The figure shows three views and two pictorial views of one solid part (mm, origin at its lowest corner). Answer the questions. A direction names the side the tool comes from. Give positions to 0.01 mm unless a question says otherwise; leave off trailing zeros. Order: outer loops, then holes, each group sorted by start corner. A loop starts at its lowest first (then second) coordinate and runs counter-clockwise, first axis right, second up. Notation, with made-up numbers: (16, 1.5) - (46, 1.5) arc R22 ccw to (46, 12.5) - close; hole circle Ø9 at (-3, -0.5). An arc over 180 degrees is marked (long way). Answer as CSV lines item,"result". Start each with the question number.
1. Section A-A on x = 170 is taken. Give the vertices of the cut face in (y, z), and give its area (3 significant figures).
2. Section D-D on y = 15.5 is taken. Give the vertices of the cut face in (x, z).
3. Section C-C on z = 8 is taken. Give the vertices of the cut face in (x, y).
4. Section B-B on y = 38.1 is taken. Give the vertices of the cut face in (x, z), and give its area (3 significant figures).
5. Which of the six approach directions +Z, -Z, +X, -X, +Y, -Y give full straight-line access (tool end or side, diameter ignored) to the marked faces 1, 2 and 3?
6. Determine the mould class of the marked faces 4, 5 and 6 for opening direction Z: +Z half, -Z half, draft (parallel to the pull), parting line (faces both ways), or undercut.
7. A flat-ended cylindrical pin translates along its axis: pin 1 (5 mm diameter, centred on y = 23, z = 61.5, fed in from +X). Find the tip coordinate at first contact, or state that the pin passes through.
8. Consider line 1 along Y through (x, z) = (170, 11); line 2 along Z through (x, y) = (84, 15.5); line 3 along X through (y, z) = (38, 86). Determine where each line is inside the solid, lowest interval first. Write a range as [from, to].
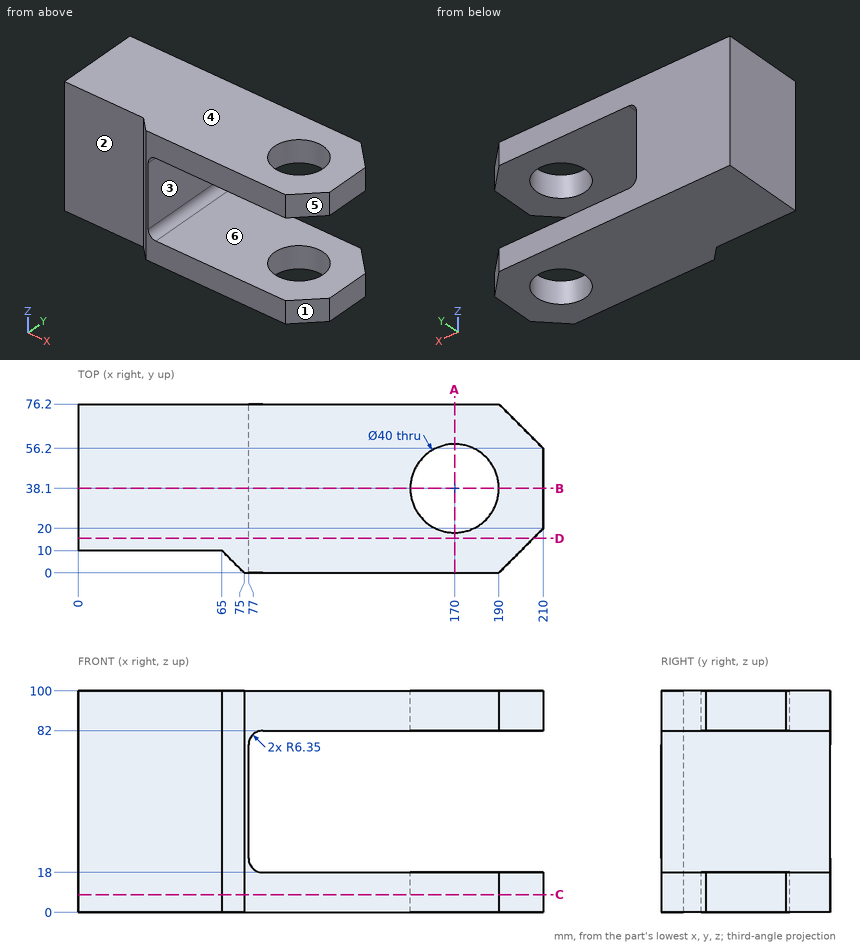
Checks:
1,outline,"(0, 0) - (18.1, 0) - (18.1, 18) - (0, 18) - close; (0, 82) - (18.1, 82) - (18.1, 100) - (0, 100) - close; (58.1, 0) - (76.2, 0) - (76.2, 18) - (58.1, 18) - close; (58.1, 82) - (76.2, 82) - (76.2, 100) - (58.1, 100) - close"
1,area,"1,300 mm²"
2,outline,"(0, 0) - (205.5, 0) - (205.5, 18) - (83.35, 18) arc R6.35 cw to (77, 24.35) - (77, 75.65) arc R6.35 cw to (83.35, 82) - (205.5, 82) - (205.5, 100) - (0, 100) - close"
3,outline,"(0, 10) - (65, 10) - (75, 0) - (190, 0) - (210, 20) - (210, 56.2) - (190, 76.2) - (0, 76.2) - close; hole circle Ø40 at (170, 38.1)"
4,outline,"(0, 0) - (150, 0) - (150, 18) - (83.35, 18) arc R6.35 cw to (77, 24.35) - (77, 75.65) arc R6.35 cw to (83.35, 82) - (150, 82) - (150, 100) - (0, 100) - close; (190, 0) - (210, 0) - (210, 18) - (190, 18) - close; (190, 82) - (210, 82) - (210, 100) - (190, 100) - close"
4,area,"11,100 mm²"
5,face 1,"+Z, -Z, +X, -Y"
5,face 2,"+Z, -Z, -X, -Y"
5,face 3,"+X, +Y, -Y"
6,face 4,"+Z half"
6,face 5,"draft"
6,face 6,"undercut"
7,pin 1,"stops at x = 77"
8,line 1,"y = [0, 18.1], [58.1, 76.2]"
8,line 2,"z = [0, 18], [82, 100]"
8,line 3,"x = [0, 150], [190, 210]"
